CAD build for the part. Positions are in the model's coordinates, mm. Face numbers are marked on the shaded views. A direction names the side the tool comes from. Round coordinates to 2 decimals unless told otherwise and drop trailing zeros. Order: outer loops, then holes, each group sorted by start corner. A loop starts at its lowest first (then second) coordinate and runs counter-clockwise, first axis right, second up. Notation, with made-up numbers: (-21, -21.5) -> (-3, -21.5) arc R15 cw to (-3, 2.5) -> close; hole circle Ø8 at (-12, 44.5). An arc over 180 degrees is marked (long way). Return JSON: item names as keys, results as strings. Group by question number.
Q1. Cut at A-A (z = 26.5). Write the cut outline in (x, y), then the cut area to 4 significant figures.
Q2. Cut at C-C (y = 0). Write the cut outline in (x, z), then the cut area to 3 significant figures.
Q3. Cut at D-D (z = 15). Write the cut outline in (x, y), then the cut area to 3 significant figures.
Q4. Probe line 1 along X through (y, z) = (33, 14.5); line 2 along Z through (x, y) = (41, 15); line 3 along Y through (x, z) = (24.5, 23.5). List the from-to ranges inside material, lowest first.
Q5. Cut at B-B (x = 0). Write the cut outline in (y, z).
Q6. Which spindle directions (+Z, -Z, +X, -X, +Y, -Y) get a long thin tool onto all of the face, cutting with end or side? Do the marked faces 1, 2 and 3. Say none if no direction does.
Q7. Flat gauge pins, fed straight in: pin 1 (15 mm diameter, centred on x = 27.5, z = 10.5, fed in from +Y); pin 2 (2.5 mm diameter, centred on x = -41.5, y = 33, fed in from -Z); pin 3 (3 mm diameter, centred on x = 19.5, y = 25.5, fed in from +Z). Where does each tip first touch, or does it go through?
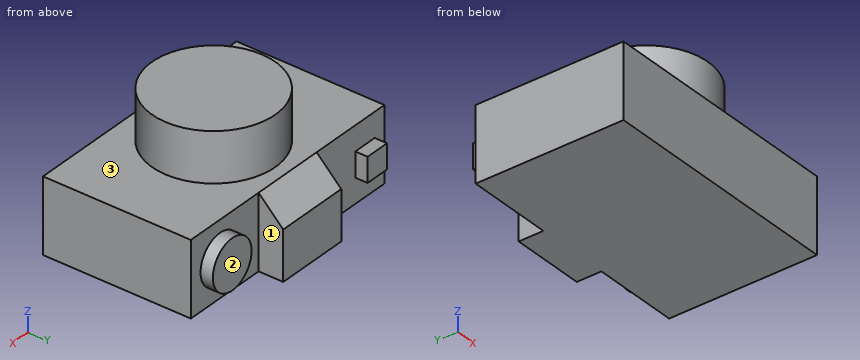
Autodesk Fusion 360 part; units mm, degrees
sketch "Sketch1" plane through (0, 0, 0) normal (0, 0, 1) x (1, 0, 0)
  line L0 (-50, 30) -> (50, 30)
  line L1 (50, 30) -> (50, -30)
  line L2 (50, -30) -> (-50, -30)
  line L3 (-50, -30) -> (-50, 30)
  dimension "d1" = 100
  dimension "d2" = 60
  dimension "d4" = 30
  dimension "d5" = 50
extrude "Extrude1" add sketch "Sketch1" along normal blind 30
sketch "Sketch2" plane through (0, 0, 30) normal (0, 0, 1) x (1, 0, 0)
  line L0 (-50, -30) -> (50, -30)
  line L1 (50, -30) -> (50, 30)
  line L2 (50, 30) -> (-50, 30)
  line L3 (-50, 30) -> (-50, -30)
  circle A0 centre (0, 0) radius 25
  dimension "d8" = 50
extrude "Extrude2" add sketch "Sketch2" along normal blind 20 contours A0
sketch "Sketch3" plane through (0, 30, 0) normal (0, 1, 0) x (-1, 0, 0)
  line L0 (-50, 0) -> (50, 0)
  line L1 (50, 0) -> (50, 30)
  line L2 (50, 30) -> (-50, 30)
  line L3 (-50, 30) -> (-50, 0)
  line L4 (15, 0) -> (-15, 0)
  line L5 (-15, 0) -> (-15, 30)
  line L6 (-15, 30) -> (15, 30)
  line L7 (15, 30) -> (15, 0)
extrude "Extrude3" add sketch "Sketch3" along normal blind 10 contours L0 L2 L4 L5 L6 L7
sketch "Sketch4" plane through (0, 30, 0) normal (0, 1, 0) x (-1, 0, 0)
  line L0 (-15, 0) -> (-15, 30)
  line L1 (-15, 30) -> (-50, 30)
  line L2 (-50, 30) -> (-50, 0)
  line L3 (-50, 0) -> (-15, 0)
  circle A0 centre (-35, 15) radius 10
  line L4 (45, 10) -> (35, 10)
  line L5 (35, 10) -> (35, 20)
  line L6 (35, 20) -> (45, 20)
  line L7 (45, 20) -> (45, 10)
  line L8 (15, 0) -> (15, 30)
  dimension "d16" = 20
  dimension "d17" = 20
  dimension "d18" = 20
extrude "Extrude4" add sketch "Sketch4" along normal blind 5 contours A0 | L4 L5 L6 L7
sketch "Sketch5" plane through (15, 0, 0) normal (1, 0, 0) x (0, 0, -1)
  line L0 (-30, 30) -> (0, 30)
  line L1 (0, 30) -> (0, 40)
  line L2 (0, 40) -> (-30, 40)
  line L3 (-30, 40) -> (-30, 30)
  line L4 (-30, 40) -> (-30, 30)
  line L5 (-30, 30) -> (-20, 40)
  line L6 (-20, 40) -> (-30, 40)
extrude "Extrude5" cut sketch "Sketch5" against normal blind 35 contours L2 L3 L4 L5 L6
sketch "Sketch6" plane through (0, 0, 50) normal (0, 0, 1) x (1, 0, 0)
  circle A0 centre (0, 0) radius 25
Solution:
{
 "1": {"outline": "(-50, -30) -> (50, -30) -> (50, 30) -> (15, 30) -> (15, 33.5) -> (-15, 33.5) -> (-15, 30) -> (-50, 30) -> close", "area": "6,105 mm²"},
 "2": {"outline": "(-50, 0) -> (50, 0) -> (50, 30) -> (25, 30) -> (25, 50) -> (-25, 50) -> (-25, 30) -> (-50, 30) -> close", "area": "4,000 mm²"},
 "3": {"outline": "(-50, -30) -> (50, -30) -> (50, 30) -> (45, 30) -> (45, 35) -> (25, 35) -> (25, 30) -> (15, 30) -> (15, 40) -> (-15, 40) -> (-15, 30) -> (-35, 30) -> (-35, 35) -> (-45, 35) -> (-45, 30) -> (-50, 30) -> close", "area": "6,450 mm²"},
 "4": {"line 1": "x = -45 to -35, -15 to 15, 25.01 to 44.99", "line 2": "z = 0 to 30", "line 3": "y = -30 to 30"},
 "5": {"outline": "(-30, 0) -> (40, 0) -> (40, 20) -> (30, 30) -> (25, 30) -> (25, 50) -> (-25, 50) -> (-25, 30) -> (-30, 30) -> close"},
 "6": {"face 1": "+Z, -Z, +Y", "face 2": "+Z, -Z, +X, +Y", "face 3": "+Z"},
 "7": {"pin 1": "stops at y = 35", "pin 2": "stops at z = 10", "pin 3": "stops at z = 30"}
}
